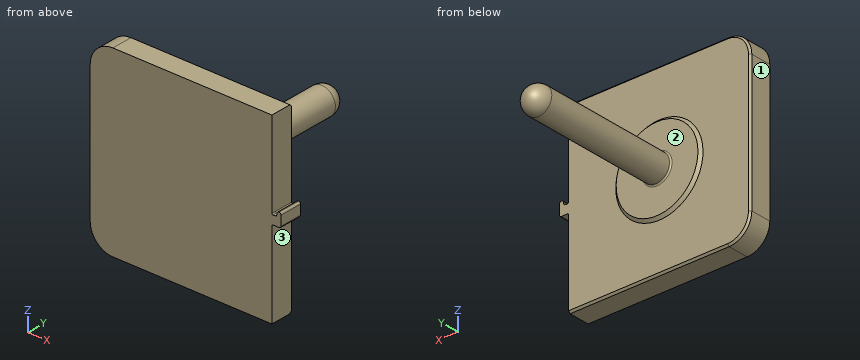
```python
from build123d import *

# Parameters (mm, degrees)
SKETCH1_W           = 200
SKETCH1_H           = 200
BOSS_EXTRUDE1_DEPTH = 25
SKETCH2_R           = 15
BOSS_EXTRUDE2_DEPTH = 170
BOSS_EXTRUDE3_DEPTH = 25
FILLET1_R           = 1
FILLET2_R           = 25
FILLET3_R           = 15
SKETCH5_R           = 45
BOSS_EXTRUDE4_DEPTH = 3
CHAMFER1_SIZE       = 3
FILLET4_R           = 1.5
CHAMFER2_SIZE       = 2


with BuildPart() as part:
    # Sketch1 → Boss-Extrude1 (new body)
    with BuildSketch(Plane(origin=(0, 0, 0), x_dir=(1, 0, 0), z_dir=(0, 1, 0))):
        Rectangle(SKETCH1_W, SKETCH1_H)
    extrude(amount=BOSS_EXTRUDE1_DEPTH)

    # Sketch2 → Boss-Extrude2 (add)
    with BuildSketch(Plane(origin=(0, 25, 0), x_dir=(1, 0, 0), z_dir=(0, 1, 0))):
        with Locations(Location((0, 0, 0), (0, 0, 270))):
            Circle(SKETCH2_R)
    extrude(amount=BOSS_EXTRUDE2_DEPTH)

    # Sketch4 → Boss-Extrude3 (add)
    with BuildSketch(Plane(origin=(0, 0, 0), x_dir=(1, 0, 0), z_dir=(0, 1, 0))):
        with BuildLine():
            Line((100, 4.8), (108, 4.8))
            ThreePointArc((108, 4.8), (109.414213562, 4.214213562), (110, 2.8))
            Line((110, 2.8), (110, -7.8))
            ThreePointArc((110, -7.8), (109.414213562, -9.214213562), (108, -9.8))
            Line((108, -9.8), (107.4, -9.8))
            ThreePointArc((107.4, -9.8), (105.985786438, -9.214213562), (105.4, -7.8))
            Line((105.4, -7.8), (105.4, -6.8))
            ThreePointArc((105.4, -6.8), (104.814213562, -5.385786438), (103.4, -4.8))
            Line((103.4, -4.8), (100, -4.8))
            Line((100, -4.8), (100, 4.8))
        make_face()
    extrude(amount=BOSS_EXTRUDE3_DEPTH)

    # Fillet1
    fillet1_edges = [part.edges().sort_by_distance(p)[0] for p in [
        (100, 12.5, -4.8),
        (100, 12.5, 4.8),
    ]]
    fillet(fillet1_edges, radius=FILLET1_R)

    # Fillet2
    fillet2_edges = [part.edges().sort_by_distance(p)[0] for p in [
        (-100, 12.5, -100),
        (-100, 12.5, 100),
    ]]
    fillet(fillet2_edges, radius=FILLET2_R)

    # Fillet3
    fillet3_edges = [part.edges().sort_by_distance(p)[0] for p in [
        (0, 195, -15),
    ]]
    fillet(fillet3_edges, radius=FILLET3_R)

    # Sketch5 → Boss-Extrude4 (add)
    with BuildSketch(Plane(origin=(0, 25, 0), x_dir=(1, 0, 0), z_dir=(0, 1, 0))):
        with Locations(Location((0, 0, 0), (0, 0, 270))):
            Circle(SKETCH5_R)
    extrude(amount=BOSS_EXTRUDE4_DEPTH)

    # Chamfer1
    chamfer1_edges = [part.edges().sort_by_distance(p)[0] for p in [
        (0, 25, -45),
    ]]
    chamfer(chamfer1_edges, length=CHAMFER1_SIZE - 0.0001)  # a hair under: the kernel refuses the full size

    # Fillet4
    fillet4_edges = [part.edges().sort_by_distance(p)[0] for p in [
        (0, 28, -15),
    ]]
    fillet(fillet4_edges, radius=FILLET4_R)

    # Chamfer2
    chamfer2_edges = [part.edges().sort_by_distance(p)[0] for p in [
        (12.5, 25, -100),
        (-100, 25, 0),
        (12.5, 25, 100),
        (-92.67766953, 25, 92.67766953),
        (-92.67766953, 25, -92.67766953),
    ]]
    chamfer(chamfer2_edges, length=CHAMFER2_SIZE)


solid = part.part
```
Check sheet for the modelled part. Datum: model origin and axes. Units: mm. Face numbers are marked on the shaded views. A direction names the side the tool comes from. Coordinates: 2 decimals unless noted, no trailing zeros. Loops run counter-clockwise (first coordinate to the right, second up) from the corner with the lowest first, then second, coordinate; pieces in that order, holes last.
1) Sectioned sample at D-D (z = -71). Record the boundary of the cut face in (x, y).
2) Sectioned sample at C-C (y = 156). Record the boundary of the cut face in (x, z).
3) Access from +Z, -Z, +X, -X, +Y, -Y to the whole of each face (thin tool, end or side, straight path). Record for the marked faces 1, 2 and 3.
4) Material ranges on probe 1 along Y at (x, z) = (-31.5, -60); probe 2 along Y at (x, z) = (27, -28.5); probe 3 along X at (y, z) = (120, -1.5), recorded low to high.
5) Gauge pin test, flat ends, axial feed: pin 1 (1.5 mm diameter, centred on x = 25.5, y = 28, fed in from +Z); pin 2 (0.7 mm diameter, centred on x = 103, y = 12, fed in from +Z); pin 3 (3 mm diameter, centred on x = -59.5, z = -71, fed in from +Y); pin 4 (3 mm diameter, centred on y = 149, z = 17, fed in from +X) (1 decimal). Record the tip position at first contact, or that the pin passes through.
Check sheet entries:
1. outline: (-100, 0) - (100, 0) - (100, 25) - (-98, 25) - (-100, 23) - close
2. outline: circle Ø30 at (0, 0)
3. face 1: +Z, -Z, -X, +Y, -Y
3. face 2: +Y
3. face 3: -Z, +X, +Y, -Y
4. probe 1: y = 0 to 25
4. probe 2: y = 0 to 28
4. probe 3: x = -14.92 to 14.92
5. pin 1: stops at z = 38.11
5. pin 2: stops at z = 4.8
5. pin 3: stops at y = 25
5. pin 4: passes through
